from build123d import *

# Parameters (mm, degrees)
BOSS_EXTRUDE1_DEPTH         = 20
M3_TAPPED_HOLE1_D           = 2.5
M3_TAPPED_HOLE1_CSINK_D     = 3.05
M3_TAPPED_HOLE1_CSINK_ANGLE = 90
M3_TAPPED_HOLE2_D           = 2.5
M3_TAPPED_HOLE2_CSINK_D     = 3.05
M3_TAPPED_HOLE2_CSINK_ANGLE = 90


with BuildPart() as part:
    # Sketch1 → Boss-Extrude1 (new body)
    with BuildSketch(Plane.XY):
        Polygon((2, 5.1), (4, 5.1), (4, 7.1), (-4, 7.1), (-4, 5.25), (-12, 5.25), (-12, 3.25), (-4, 3.25), (-4, -9.9), (4, -9.9), (4, -7.9), (2, -7.9), (-2, -7.9), (-2, 5.1), align=None)
    extrude(amount=BOSS_EXTRUDE1_DEPTH)

    # M3 Tapped Hole1 (through all)
    with Locations(Plane(origin=(-8.108371913, 5.25, 4), x_dir=(1, 0, 0), z_dir=(0, 1, 0))):
        with Locations((0, 0), (0, -12)):
            CounterSinkHole(M3_TAPPED_HOLE1_D / 2, M3_TAPPED_HOLE1_CSINK_D / 2, counter_sink_angle=M3_TAPPED_HOLE1_CSINK_ANGLE)

    # M3 Tapped Hole2 (through all)
    with Locations(Plane(origin=(1.2, 7.1, 10), x_dir=(0, 0, 1), z_dir=(0, 1, 0))):
        with Locations((0, 0)):
            CounterSinkHole(M3_TAPPED_HOLE2_D / 2, M3_TAPPED_HOLE2_CSINK_D / 2, counter_sink_angle=M3_TAPPED_HOLE2_CSINK_ANGLE)


solid = part.part
Geometry check sheet. Reference: the model listing, model coordinates, mm. A direction names the side the tool comes from. Round coordinates to 2 decimals unless told otherwise and drop trailing zeros. Loops run counter-clockwise (first coordinate to the right, second up) from the corner with the lowest first, then second, coordinate; pieces in that order, holes last. Notation, with made-up numbers: (28.25, -40) -> (33.25, -40) arc R36 ccw to (33.25, -1) -> close; hole circle Ø7 at (59, 46). An arc over 180 degrees is marked (long way). Answer as a JSON object with one key per item and string values. Group by question number.
Item 1: Cross-section at C-C, the plane z = 10. Record the cut outline in (x, y) (3 decimals), plus the area to 3 significant figures.
Item 2: Cross-section at D-D, the plane z = 6. Record the cut outline in (x, y), plus the area to 3 significant figures.
Item 3: Set-up check for faces 1 (the face through (1.25, -8.91, 11.25)), 2 (the face through (-0.3, -7.9, 9.9)), 3 (the face through (-4, -3, 10)), 4 (the face through (-4, 6, 10)): record each of +Z, -Z, +X, -X, +Y, -Y from which the full face is reachable in a straight line by a thin tool's end or side.
Item 4: Depth check by flat-ended pin: pin 1 Ø9 at (x, z) = (-10, 10.5) entering from +Y; pin 2 Ø2 at (y, z) = (6.5, 13) entering from -X; pin 3 Ø3 at (x, z) = (-8.11, 16) entering from -Y. Enter the tip coordinate at first touch or a pass-through.
Item 5: Cross-section at B-B, the plane z = 4. Record the cut outline in (x, y) (3 decimals).
Item 6: Release check for a two-part mould opening along Y. For faces 5 (the face through (-0.4, 5.1, 9.9)), 6 (the face through (-8, 3.25, 10)), 7 (the face through (-3, -1, 20)) record: pulls with the +Y half, pulls with the -Y half, needs draft (parallel to the pull), parting line crosses it, or undercut.
Item 7: Thickness scan on line 1 along Z through (x, y) = (1.2, 6.55); line 2 along Y through (x, z) = (2.5, 11.25); line 3 along Y through (x, z) = (-6.25, 16.75). Record the ranges inside material, lowest first.
Item 8: Cross-section at A-A, the plane x = 1.2. Record the cut outline in (y, z) (3 decimals).
Determined:
{
 "1": {"outline": "(-12, 3.25) -> (-4, 3.25) -> (-4, -9.9) -> (-0.05, -9.9) -> (-0.05, -7.9) -> (-2, -7.9) -> (-2, 5.1) -> (-0.05, 5.1) -> (-0.05, 6.825) -> (-0.325, 7.1) -> (-4, 7.1) -> (-4, 5.25) -> (-12, 5.25) -> close; (2.45, -9.9) -> (4, -9.9) -> (4, -7.9) -> (2.45, -7.9) -> close; (2.45, 5.1) -> (4, 5.1) -> (4, 7.1) -> (2.725, 7.1) -> (2.45, 6.825) -> close", "area": "63.9 mm²"},
 "2": {"outline": "(-12, 3.25) -> (-4, 3.25) -> (-4, -9.9) -> (4, -9.9) -> (4, -7.9) -> (-2, -7.9) -> (-2, 5.1) -> (4, 5.1) -> (4, 7.1) -> (-4, 7.1) -> (-4, 5.25) -> (-12, 5.25) -> close", "area": "74.0 mm²"},
 "3": {"face 1": "+Y, -Y", "face 2": "+Z, -Z, +X", "face 3": "+Z, -Z, -X, -Y", "face 4": "+Z, -Z, -X, +Y"},
 "4": {"pin 1": "stops at y = 5.25", "pin 2": "stops at x = -4", "pin 3": "stops at y = 3.25"},
 "5": {"outline": "(-12, 3.25) -> (-9.358, 3.25) -> (-9.358, 4.975) -> (-9.633, 5.25) -> (-12, 5.25) -> close; (-6.858, 3.25) -> (-4, 3.25) -> (-4, -9.9) -> (4, -9.9) -> (4, -7.9) -> (-2, -7.9) -> (-2, 5.1) -> (4, 5.1) -> (4, 7.1) -> (-4, 7.1) -> (-4, 5.25) -> (-6.583, 5.25) -> (-6.858, 4.975) -> close"},
 "6": {"face 5": "undercut", "face 6": "pulls with the -Y half", "face 7": "needs draft"},
 "7": {"line 1": "z = 0 to 8.75, 11.25 to 20", "line 2": "y = -9.9 to -7.9, 5.1 to 7.1", "line 3": "y = 3.25 to 5.25"},
 "8": {"outline": "(-9.9, 0) -> (-7.9, 0) -> (-7.9, 8.75) -> (-9.9, 8.75) -> close; (-9.9, 11.25) -> (-7.9, 11.25) -> (-7.9, 20) -> (-9.9, 20) -> close; (5.1, 0) -> (7.1, 0) -> (7.1, 8.475) -> (6.825, 8.75) -> (5.1, 8.75) -> close; (5.1, 11.25) -> (6.825, 11.25) -> (7.1, 11.525) -> (7.1, 20) -> (5.1, 20) -> close"}
}
